from build123d import *

# Parameters (mm, degrees)
BOSS_EXTRUDE3_DEPTH = 1.905
BOSS_EXTRUDE4_DEPTH = 86.995
CUT_EXTRUDE2_DEPTH  = 85.09
SKETCH16_W          = 82.55
SKETCH16_H          = 85.09
CUT_EXTRUDE3_DEPTH  = 86.36
SKETCH18_W          = 80.01
SKETCH18_H          = 85.09
CUT_EXTRUDE4_DEPTH  = 86.36
SKETCH19_R          = 6.35
BOSS_EXTRUDE5_DEPTH = 86.36
CUT_EXTRUDE5_REACH  = 90.9
SKETCH20_R          = 11.2395
SKETCH20_R_2        = 1.5875


with BuildPart() as part:
    # Sketch7 → Boss-Extrude3 (new body)
    with BuildSketch(Plane(origin=(0, 0, 0), x_dir=(1, 0, 0), z_dir=(0, 1, 0))):
        with BuildLine():
            Line((-38.1, 44.45), (38.1, 44.45))
            ThreePointArc((38.1, 44.45), (42.590128061, 42.590128061), (44.45, 38.1))
            Line((44.45, 38.1), (44.45, -38.1))
            ThreePointArc((44.45, -38.1), (42.590128061, -42.590128061), (38.1, -44.45))
            Line((38.1, -44.45), (-38.1, -44.45))
            ThreePointArc((-38.1, -44.45), (-42.590128061, -42.590128061), (-44.45, -38.1))
            Line((-44.45, -38.1), (-44.45, 38.1))
            ThreePointArc((-44.45, 38.1), (-42.590128061, 42.590128061), (-38.1, 44.45))
        make_face()
    extrude(amount=BOSS_EXTRUDE3_DEPTH)

    # Sketch7_2 → Boss-Extrude4 (add)
    with BuildSketch(Plane(origin=(0, 0, 0), x_dir=(1, 0, 0), z_dir=(0, 1, 0))):
        with BuildLine():
            Line((-38.1, 44.45), (38.1, 44.45))
            ThreePointArc((38.1, 44.45), (42.590128061, 42.590128061), (44.45, 38.1))
            Line((44.45, 38.1), (44.45, -38.1))
            ThreePointArc((44.45, -38.1), (42.590128061, -42.590128061), (38.1, -44.45))
            Line((38.1, -44.45), (-38.1, -44.45))
            ThreePointArc((-38.1, -44.45), (-42.590128061, -42.590128061), (-44.45, -38.1))
            Line((-44.45, -38.1), (-44.45, 38.1))
            ThreePointArc((-44.45, 38.1), (-42.590128061, 42.590128061), (-38.1, 44.45))
        make_face()
    extrude(amount=-BOSS_EXTRUDE4_DEPTH)

    # Sketch15 → Cut-Extrude2 (cut)
    with BuildSketch(Plane(origin=(0, 0, 0), x_dir=(1, 0, 0), z_dir=(0, 1, 0))):
        with BuildLine():
            Line((-35.56, 41.91), (35.56, 41.91))
            ThreePointArc((35.56, 41.91), (40.050128061, 40.050128061), (41.91, 35.56))
            Line((41.91, 35.56), (41.91, -35.56))
            ThreePointArc((41.91, -35.56), (40.050128061, -40.050128061), (35.56, -41.91))
            Line((35.56, -41.91), (-35.56, -41.91))
            ThreePointArc((-35.56, -41.91), (-40.050128061, -40.050128061), (-41.91, -35.56))
            Line((-41.91, -35.56), (-41.91, 35.56))
            ThreePointArc((-41.91, 35.56), (-40.050128061, 40.050128061), (-35.56, 41.91))
        make_face()
    extrude(amount=-CUT_EXTRUDE2_DEPTH, mode=Mode.SUBTRACT)

    # Sketch16 → Cut-Extrude3 (cut)
    with BuildSketch(Plane.XY.offset(44.45)):
        with Locations((-3.175, -42.545)):
            Rectangle(SKETCH16_W, SKETCH16_H)
    extrude(amount=-CUT_EXTRUDE3_DEPTH, mode=Mode.SUBTRACT)

    # Sketch18 → Cut-Extrude4 (cut)
    with BuildSketch(Plane.ZY.offset(-41.91)):
        with Locations((4.445, -42.545)):
            Rectangle(SKETCH18_W, SKETCH18_H)
    extrude(amount=CUT_EXTRUDE4_DEPTH, mode=Mode.SUBTRACT)

    # Sketch19 → Boss-Extrude5 (add)
    with BuildSketch(Plane(origin=(0, -85.09, 0), x_dir=(1, 0, 0), z_dir=(0, 1, 0))):
        with Locations((-38.1, -38.1)):
            Circle(SKETCH19_R)
    extrude(amount=BOSS_EXTRUDE5_DEPTH)

    # Sketch20 → Cut-Extrude5 (cut, up to next)
    with BuildSketch(Plane(origin=(0, 1.905, 0), x_dir=(1, 0, 0), z_dir=(0, 1, 0)), mode=Mode.PRIVATE) as cut_extrude5_sk1:
        Circle(SKETCH20_R)
    cut_extrude5_tool1 = extrude(cut_extrude5_sk1.sketch, amount=-CUT_EXTRUDE5_REACH, mode=Mode.PRIVATE) & part.part
    add(cut_extrude5_tool1.solids().sort_by_distance((0, 1.905, 0))[0], mode=Mode.SUBTRACT)
    # Sketch20 → Cut-Extrude5 (cut, up to next)
    with BuildSketch(Plane(origin=(0, 1.905, 0), x_dir=(1, 0, 0), z_dir=(0, 1, 0)), mode=Mode.PRIVATE) as cut_extrude5_sk2:
        with Locations((-15.875, 0)):
            Circle(SKETCH20_R_2)
    cut_extrude5_tool2 = extrude(cut_extrude5_sk2.sketch, amount=-CUT_EXTRUDE5_REACH, mode=Mode.PRIVATE) & part.part
    add(cut_extrude5_tool2.solids().sort_by_distance((-15.875, 1.905, 0))[0], mode=Mode.SUBTRACT)
    # Sketch20 → Cut-Extrude5 (cut, up to next)
    with BuildSketch(Plane(origin=(0, 1.905, 0), x_dir=(1, 0, 0), z_dir=(0, 1, 0)), mode=Mode.PRIVATE) as cut_extrude5_sk3:
        with Locations((15.875, 0)):
            Circle(SKETCH20_R_2)
    cut_extrude5_tool3 = extrude(cut_extrude5_sk3.sketch, amount=-CUT_EXTRUDE5_REACH, mode=Mode.PRIVATE) & part.part
    add(cut_extrude5_tool3.solids().sort_by_distance((15.875, 1.905, 0))[0], mode=Mode.SUBTRACT)


solid = part.part
Here's how the part is built. I have some questions about the finished solid (model axes, mm). A direction names the side the tool comes from. Coordinates: 2 decimals unless noted, no trailing zeros. Loops run counter-clockwise (first coordinate to the right, second up) from the corner with the lowest first, then second, coordinate; pieces in that order, holes last.
1. If we mould it in two halves opening along Z, with no side actions, what happens to faces 3 (the cylindrical face through (40.844, -41.949, -39.081)), 4 (the flat face through (11, 1.905, -11)), 5 (the cylindrical face through (-17.46, 0.97, -0.07)), 6 (the cylindrical face through (-1.463, 0.966, -11.144))? For each: pulls with the +Z half, pulls with the -Z half, needs draft (parallel to the pull), parting line crosses it, or undercut.
2. Imagine slicing it at B-B, the plane y = -41.5. Please give me the cut outline in (x, z), and give its area (3 significant figures).
3. I need wall thicknesses on L1, parallel to X at y = 0.65, z = 0; L2, parallel to Y at x = -37.5, z = -4 (3 decimals); L3, parallel to Z at x = -38, y = -17. Which ranges of each line are inside material? Lowest first, please.
4. For P1, Ø12, axis at x = 3, y = -66, coming from the +Z side; P2, Ø20, axis at x = 0, z = 0, coming from the +Y side; P3, Ø4, axis at y = -60.5, z = -34.5, coming from the -X side, each with a flat end and sliding along its axis, tell me the tip position at first contact or that it passes through.
5. For faces 1 (the flat face through (1, -86.995, -1)), 2 (the cylindrical face through (14.29, 0.97, -0.07)), which set-ups out of +Z, -Z, +X, -X, +Y, -Y let a thin tool reach every point of the face, with its end or its side?
6. Imagine slicing it at D-D, the plane z = 16. Please give me the cut outline in (x, y) (3 decimals).
7. Imagine slicing it at A-A, the plane z = 0. Count the separate pieces of the cut face and the enclosed holes in it, and give its area (3 significant figures).
Taken from the geometry:
1. face 3: pulls with the +Z half
1. face 4: needs draft
1. face 5: undercut
1. face 6: undercut
2. outline: circle Ø12.7 at (-38.1, 38.1); (-43.18, -41.91) arc R6.35 ccw to (-38.1, -44.45) - (38.1, -44.45) arc R6.35 ccw to (44.45, -38.1) - (44.45, 38.1) arc R6.35 ccw to (41.91, 43.18) - (41.91, -35.56) arc R6.35 cw to (38.1, -41.38) - (38.1, -41.91) - close
2. area: 557 mm2
3. L1: x = -44.45 to -17.46, -14.29 to -11.24, 11.24 to 14.29, 17.46 to 44.45
3. L2: y = -86.995 to -85.09, 0 to 1.905
3. L3: z = -44.45 to -41.91, 31.75 to 44.45
4. P1: stops at z = -41.91
4. P2: stops at y = -85.09
4. P3: stops at x = 41.84
5. face 1: +Z, -Z, +X, -X, -Y
5. face 2: +Y
6. outline: (-44.45, -86.995) - (44.45, -86.995) - (44.45, 1.905) - (-44.45, 1.905) - (-44.45, 0) - (41.91, 0) - (41.91, -85.09) - (-44.45, -85.09) - close
7. separate pieces: 4
7. enclosed holes: 0
7. area: 500 mm2
